from build123d import *

# Parameters (mm, degrees)
F0_R      = 13.75
F1_DEPTH  = 40.5
F2_R      = 16
F3_DEPTH  = 33.6
F4_R      = 10
F5_DEPTH  = 3
F6_R      = 3
F7_DEPTH  = 17
F8_W      = 9.724755
F8_H      = 3.28539
F9_DEPTH  = 12
F10_R     = 1.5
F11_DEPTH = 5.5


with BuildPart() as f1:
    # F0 (on Right) → F1 (new body)
    with BuildSketch(Plane.YZ):
        Circle(F0_R)
    extrude(amount=F1_DEPTH)

    # F2 (on face) → F3 (join)
    with BuildSketch(Plane.YZ.offset(40.5)):
        Circle(F2_R)
    extrude(amount=F3_DEPTH)

    # F4 (on face) → F5 (join)
    with BuildSketch(Plane.YZ.offset(74.1)):
        Circle(F4_R)
    extrude(amount=F5_DEPTH)

    # F6 (on face) → F7 (join)
    with BuildSketch(Plane.YZ.offset(77.1)):
        Circle(F6_R)
    extrude(amount=F7_DEPTH)

    # F8 (on face) → F9 (cut)
    with BuildSketch(Plane.YZ.offset(94.1)):
        with Locations((0.085164, 4.142695)):
            Rectangle(F8_W, F8_H)
    extrude(amount=-F9_DEPTH, mode=Mode.SUBTRACT)

    # F10 (on face) → F11 (cut)
    with BuildSketch(Plane.YZ.offset(74.1)):
        with Locations((0, 13)):
            Circle(F10_R)
        with Locations((13, 0)):
            Circle(F10_R)
        with Locations((0, -13)):
            Circle(F10_R)
        with Locations((-13, 0)):
            Circle(F10_R)
    extrude(amount=-F11_DEPTH, mode=Mode.SUBTRACT)


solid = f1.part
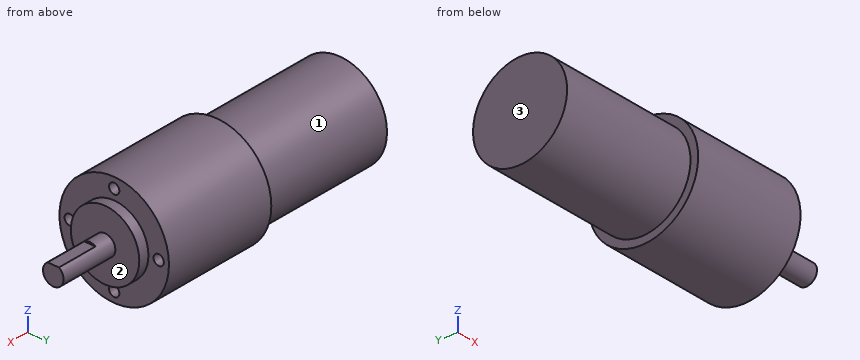
Input: part model. Units: mm. Frame: model coordinates. Face numbers are marked on the shaded views. A direction names the side the tool comes from. Coordinates: 2 decimals unless noted, no trailing zeros. Loops run counter-clockwise (first coordinate to the right, second up) from the corner with the lowest first, then second, coordinate; pieces in that order, holes last. Notation, with made-up numbers: (85, 83.25) -> (118, 83.25) arc R30 ccw to (118, 110.25) -> close; hole circle Ø11 at (35, 68). An arc over 180 degrees is marked (long way). One line per item, written item: value.
(1) Pin query (flat end, axial travel): pin 1 Ø2.5 at (x, y) = (85, 0) entering from +Z; pin 2 Ø1.5 at (y, z) = (4, -2.5) entering from +X; pin 3 Ø2.5 at (y, z) = (12.5, 0.5) entering from +X. Return the tip coordinate at first contact, or that it passes through.
Answer below:
pin 1: stops at z = 2.5
pin 2: stops at x = 77.1
pin 3: stops at x = 74.1
(2) Ray query, line 1 along Z through (x, y) = (72, 0); line 2 along X through (y, z) = (2, -4.5); line 3 along X through (y, z) = (2.5, 11.5). Return the intervals inside material, ascending.
Answer below:
line 1: z = -16 to -14.5, -11.5 to 11.5, 14.5 to 16
line 2: x = 0 to 77.1
line 3: x = 0 to 74.1
(3) Cut plane D-D (x = 7). Output: boundary loops of the cut face in (y, z).
Answer below:
outline: circle Ø27.5 at (0, 0)
(4) Cut plane C-C (x = 87). Output: boundary loops of the cut face in (y, z).
Answer below:
outline: (-1.66, 2.5) arc R3 ccw (long way) to (1.66, 2.5) -> close
(5) Set-up query: the marked faces 1, 2 and 3. Return all of +Z, -Z, +X, -X, +Y, -Y with unobstructed straight access to the full face (end or side cutting, diameter ignored); none if empty.
Answer below:
face 1: -X
face 2: +X
face 3: +Z, -Z, -X, +Y, -Y
(6) Cut plane B-B (z = 0). Output: boundary loops of the cut face in (x, y).
Answer below:
outline: (0, -13.75) -> (40.5, -13.75) -> (40.5, -16) -> (74.1, -16) -> (74.1, -14.5) -> (68.6, -14.5) -> (68.6, -11.5) -> (74.1, -11.5) -> (74.1, -10) -> (77.1, -10) -> (77.1, -3) -> (94.1, -3) -> (94.1, 3) -> (77.1, 3) -> (77.1, 10) -> (74.1, 10) -> (74.1, 11.5) -> (68.6, 11.5) -> (68.6, 14.5) -> (74.1, 14.5) -> (74.1, 16) -> (40.5, 16) -> (40.5, 13.75) -> (0, 13.75) -> close
(7) Cut plane A-A (y = 0). Output: boundary loops of the cut face in (x, z), then the cut area to 3 significant figures.
Answer below:
outline: (0, -13.75) -> (40.5, -13.75) -> (40.5, -16) -> (74.1, -16) -> (74.1, -14.5) -> (68.6, -14.5) -> (68.6, -11.5) -> (74.1, -11.5) -> (74.1, -10) -> (77.1, -10) -> (77.1, -3) -> (94.1, -3) -> (94.1, 2.5) -> (82.1, 2.5) -> (82.1, 3) -> (77.1, 3) -> (77.1, 10) -> (74.1, 10) -> (74.1, 11.5) -> (68.6, 11.5) -> (68.6, 14.5) -> (74.1, 14.5) -> (74.1, 16) -> (40.5, 16) -> (40.5, 13.75) -> (0, 13.75) -> close
area: 2,310 mm2
